Study the drawing (mm; zero at the part's minimum x, y, z) and answer. Round coordinates to 2 decimals unless told otherwise and drop trailing zeros. Order: outer loops, then holes, each group sorted by start corner. A loop starts at its lowest first (then second) coordinate and runs counter-clockwise, first axis right, second up. Notation, with made-up numbers: M -29.5,16.5 L 24.5,16.5 A22 ccw 24.5,25.5 Z; hole C 67,38 d8. An arc over 180 degrees is marked long. Put each result on its own line as item: value. Start each with the question number.
1. The part is cut by section A-A (z = 22). Give the vertices of the cut face in (x, y).
2. The part is cut by section D-D (x = 11). Give the vertices of the cut face in (y, z).
3. Consider line 1 (Y direction, x = 8, z = 14); line 2 (X direction, y = 6.5, z = 42); line 3 (Y direction, x = 7.25, z = 40.5) (1 decimal). Determine where each line is inside the solid, lowest interval first.
4. Each of these flat-tipped pins is pushed along its axis until it touches: pin 1 Ø6.5 at (x, y) = (8, 8) entering from -Z; pin 2 Ø3 at (x, z) = (11, 34) entering from -Y; pin 3 Ø2 at (y, z) = (9.5, 31) entering from -X; pin 4 Ø1.5 at (x, z) = (10, 29) entering from +Y. Where does it stop, or does it pass through?
5. The part is cut by section C-C (y = 2.75). Give the vertices of the cut face in (x, z), then the cut area to 3 significant figures.
6. The part is cut by section B-B (z = 38.5). Give the vertices of the cut face in (x, y).
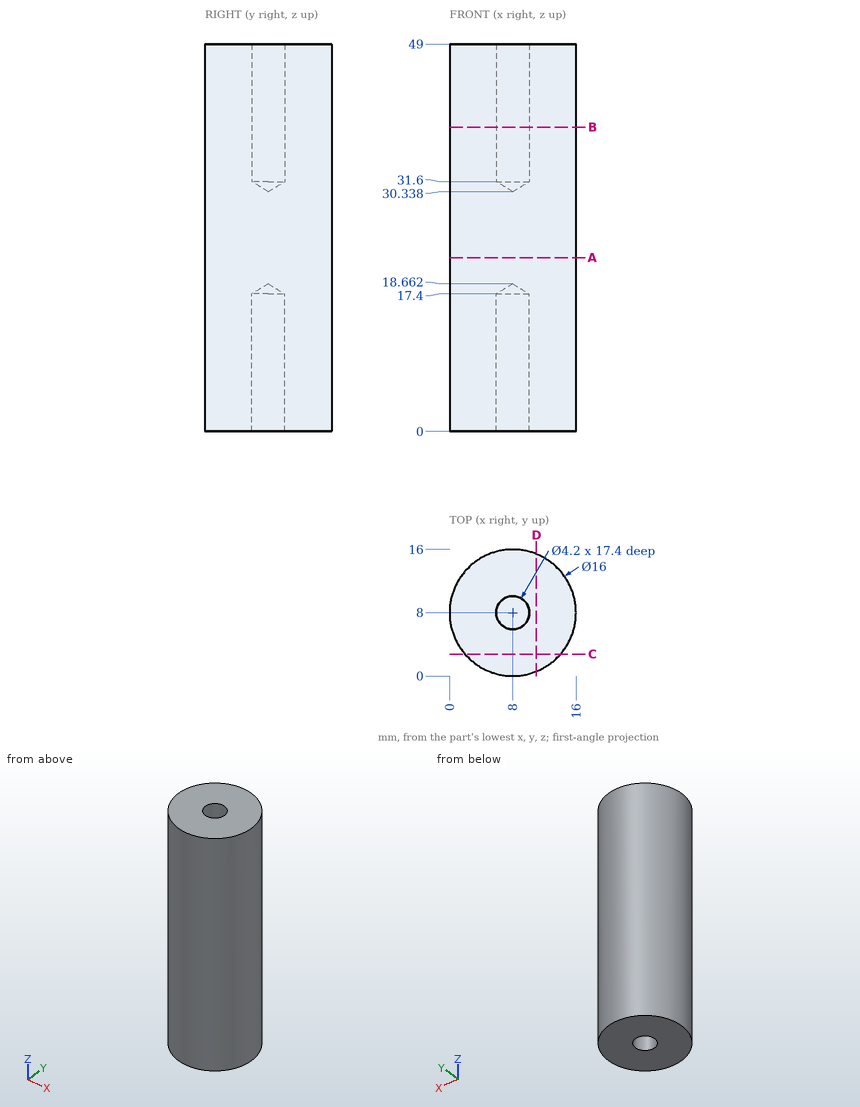
Resolved:
1. outline: C 8,8 d16
2. outline: M 0.58,0 L 15.42,0 L 15.42,49 L 0.58,49 Z
3. line 1: 0 to 5.9, 10.1 to 16
3. line 2: 0.14 to 6.53, 9.47 to 15.86
3. line 3: 0 to 6, 10 to 16
4. pin 1: z = 0
4. pin 2: y = 0.14
4. pin 3: x = 0.02
4. pin 4: y = 15.9
5. outline: M 1.96,0 L 14.04,0 L 14.04,49 L 1.96,49 Z
5. area: 592 mm2
6. outline: C 8,8 d16; hole C 8,8 d4.2
